```python
from build123d import *

# Parameters (mm, degrees)
F1_DEPTH       = 214.3125
F2_R           = 0.635
F4_D           = 3.3
F4_DEPTH       = 14.4876
F4_CBORE_D     = 6.5
F4_CBORE_DEPTH = 3
F4_TIP         = 0.9914200214
F5_DEPTH       = 0.508
F6_DEPTH       = 0.508


with BuildPart() as f1:
    # F0 (on Front) → F1 (new body)
    with BuildSketch(Plane.XZ):
        Polygon((-9.5129261665, 6.35), (-9.5129261665, 0), (3.1870738335, 0), (3.1870738335, 6.35), (1.0164155129, 6.35), (1.0164155129, 8.89), (3.1870738335, 8.89), (3.1870738335, 12.7), (-9.5129261665, 12.7), (-9.5129261665, 8.89), (-7.3422678459, 8.89), (-7.3422678459, 6.35), align=None)
    extrude(amount=F1_DEPTH)

    # F2
    f2_edges = [f1.edges().sort_by_distance(p)[0] for p in [
        (3.187074, -107.15625, 8.89),
        (-9.512926, -107.15625, 8.89),
        (-7.342268, -107.15625, 8.89),
        (-7.342268, -107.15625, 6.35),
        (-9.512926, -107.15625, 6.35),
        (1.016416, -107.15625, 6.35),
        (3.187074, -107.15625, 6.35),
        (1.016416, -107.15625, 8.89),
        (3.187074, -107.15625, 12.7),
        (-9.512926, -107.15625, 12.7),
        (-9.512926, -107.15625, 0),
        (3.187074, -107.15625, 0),
    ]]
    fillet(f2_edges, radius=F2_R)

    # F4
    with Locations(Plane.XY.offset(12.7)):
        with Locations((-3.1629261665, -30.95625), (-3.1629261665, -81.75625), (-3.1629261665, -132.55625), (-3.1629261665, -183.35625)):
            CounterBoreHole(F4_D / 2, F4_CBORE_D / 2, F4_CBORE_DEPTH, depth=F4_DEPTH)
            with Locations((0, 0, -(F4_DEPTH + F4_TIP / 2))):  # 118° drill point
                Cone(0, F4_D / 2, F4_TIP, mode=Mode.SUBTRACT)

    # F5 (cut): a face of the model
    f5_faces = [f1.faces().sort_by_distance(p)[0] for p in [
        (-3.1629261665, -214.3125, 6.2565868028),
    ]]
    extrude(f5_faces, amount=-F5_DEPTH, mode=Mode.SUBTRACT)

    # F6 (cut): a face of the model
    f6_faces = [f1.faces().sort_by_distance(p)[0] for p in [
        (-3.1629261665, 0, 6.2565868028),
    ]]
    extrude(f6_faces, amount=-F6_DEPTH, mode=Mode.SUBTRACT)


solid = f1.part
```
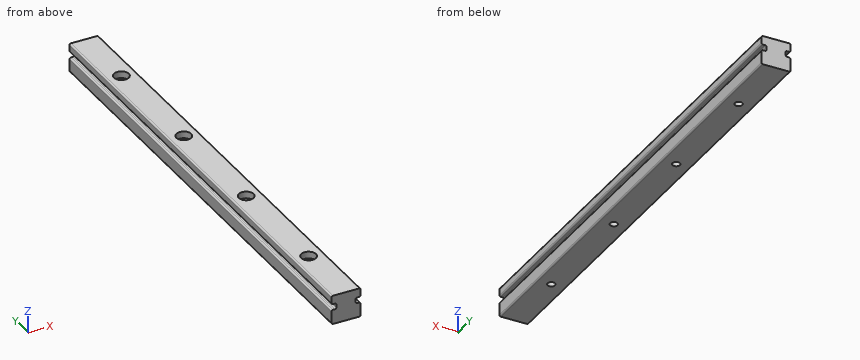
Could you check a few things on this model? Use its own coordinates, in mm. Round coordinates to 2 decimals unless told otherwise and drop trailing zeros. Write each loop counter-clockwise with the first axis right and the second up, starting at its lowest first coordinate (ties: lowest second). Pieces come first, ordered by that corner, then holes. Notation, with made-up numbers: M 26,-23.75 L 44,-23.75 A25 ccw 44,-1.75 Z; hole C 13.5,75 d9. An arc over 180 degrees is marked long. Answer in a Markdown table with one row per item. Add a question column.
Q1. If I drill on line 1 (Y direction, x = -2.5, z = 2.5); line 2 (Z direction, x = 1.5, y = -195); line 3 (Y direction, x = -4.5, z = 4), over which ranges is the centre line in solid material (lowest first)? Write a range as from..to.
Q2. Will these pins go through, and if not, where does the flat tip stop? pin 1 Ø2 at (x, y) = (-3.16, -81.76) entering from -Z; pin 2 Ø4 at (x, y) = (-3.16, -132.56) entering from +Z; pin 3 Ø1.5 at (y, z) = (-170, 8) entering from -X.
Q3. Imagine slicing it at A-A (y = -113). Please give me the cut outline in (x, z) (3 decimals), then the cut area to 3 significant figures.
Values:
| question | item | result |
|---|---|---|
| 1 | line 1 | -213.8..-184.87, -181.85..-134.07, -131.05..-83.27, -80.25..-32.47, -29.45..-0.51 |
| 1 | line 2 | 0..6.37, 8.87..12.7 |
| 1 | line 3 | -213.8..-184.32, -182.39..-133.52, -131.59..-82.72, -80.79..-31.92, -29.99..-0.51 |
| 2 | pin 1 | through |
| 2 | pin 2 | z = 9.7 |
| 2 | pin 3 | x = -7.58 |
| 3 | outline | M -9.513,0.635 A0.635 ccw -8.878,0 L 2.552,0 A0.635 ccw 3.187,0.635 L 3.187,5.715 A0.635 ccw 2.552,6.35 L 1.651,6.35 A0.635 cw 1.016,6.985 L 1.016,8.255 A0.635 cw 1.651,8.89 L 2.552,8.89 A0.635 ccw 3.187,9.525 L 3.187,12.065 A0.635 ccw 2.552,12.7 L -8.878,12.7 A0.635 ccw -9.513,12.065 L -9.513,9.525 A0.635 ccw -8.878,8.89 L -7.977,8.89 A0.635 cw -7.342,8.255 L -7.342,6.985 A0.635 cw -7.977,6.35 L -8.878,6.35 A0.635 ccw -9.513,5.715 Z |
| 3 | area | 150 mm^2 |
